Autodesk Inventor part; units mm, degrees
ref_plane "YZ Plane" through (0, 0, 0) normal (1, 0, 0) x (0, 1, 0)
ref_plane "XZ Plane" through (0, 0, 0) normal (0, 1, 0) x (-1, 0, 0)
ref_plane "XY Plane" through (0, 0, 0) normal (0, 0, 1) x (1, 0, 0)
ref_plane "Work Plane1" through (0, 0, 0) normal (0, 0, 1) x (1, 0, 0)
ref_plane "Work Plane2" through (0, 0, -10) normal (0, 0, 1) x (1, 0, 0)
sketch "Sketch1" plane through (0, 0, -10) normal (0, 0, 1) x (1, 0, 0)
  circle A0 centre (14.95, 17.4977) radius 7.15
  line L0 (0, 2.471) -> (29.9, 2.471)
  line L1 (0, 2.471) -> (0, 18.471)
  line L2 (0, 18.471) -> (-2, 18.471)
  line L3 (-2, 18.471) -> (-2, -1.5)
  line L4 (29.9, -1.5) -> (-2, -1.5)
  line L5 (29.9, -1.5) -> (29.9, 2.471)
  line L6 (4.95, 2.471) -> (24.95, 2.471)
  line L7 (24.95, 2.471) -> (24.95, 27.471)
  line L8 (24.95, 27.471) -> (4.95, 27.471)
  line L9 (4.95, 27.471) -> (4.95, 2.471)
  circle A1 centre (14.95, 17.4977) radius 8.1
  point P0 (0, 0)
  dimension "d6" = 20
  dimension "d7" = 25
  dimension "d8" = 10
  dimension "d23" = 16.2
extrude "Extrusion1" add sketch "Sketch1" against normal blind 30 contours L9 L8 L7 L0
sketch "Sketch2" plane through (4.95, 2.471, -10) normal (0, -1, 0) x (1, 0, 0)
  circle A0 centre (18.15, -13.73) radius 2.45
  circle A1 centre (1.85, -13.73) radius 2.75
  circle A2 centre (18.15, -13.73) radius 1.45
  circle A3 centre (1.85, -13.73) radius 1.45
  point P0 (-4.95, 10)
  dimension "d10" = 2.9
  dimension "d11" = 2.9
extrude "Extrusion2" cut sketch "Sketch2" against normal through all contours A2 | A3
chamfer "Chamfer1" distance 7 angle 45 2 edges at (24.95, 27.471, -25) (4.95, 27.471, -25)
sketch "Sketch3" plane through (11.95, 27.471, -10) normal (0, 1, 0) x (1, 0, 0)
  line L0 (0, 0) -> (0, 30)
  line L1 (6, 0) -> (0, 0)
  line L2 (6, 30) -> (6, 0)
  line L3 (0, 30) -> (6, 30)
  circle A0 centre (2, 5.2757) radius 1.45
  circle A1 centre (2, 26.8475) radius 1.45
  point P0 (-11.95, -10)
  dimension "d17" = 2.9
  dimension "d18" = 2.9
extrude "Extrusion3" cut sketch "Sketch3" against normal blind 10 contours A0 | A1
ref_plane "Work Plane3" through (0, 27.471, -10) normal (0, -0.7071068, 0.7071068) x (1, 0, 0)
ref_plane "Work Plane4" through (11.95, 27.471, -10) normal (0, 0.7071068, 0.7071068) x (1, 0, 0)
ref_plane "Work Plane5" through (14.95, 2.471, -10) normal (1, 0, 0) x (0, 0, -1)
sketch "Sketch5" plane through (14.95, 2.471, -10) normal (1, 0, 0) x (0, 0, -1)
  line L0 (0, 23.1268) -> (30, 23.1268)
  line L1 (0, 6.9268) -> (30, 6.9268)
  line L2 (0, 23.1268) -> (-4.2183, 23.1268)
  line L3 (-4.2183, 23.1268) -> (24.7731, 52.1181)
  line L4 (24.7731, 52.1181) -> (24.7731, 23.1268)
  point P0 (-10, -2.471)
  dimension "d21" = 41
  dimension "d22" = 45
properties part number "cellSTORM_v5_bluelaser_adapter"
Can you work these out from the model? Positions are in its coordinate system, mm. A direction names the side the tool comes from. Round coordinates to 2 decimals unless told otherwise and drop trailing zeros. Loops run counter-clockwise (first coordinate to the right, second up) from the corner with the lowest first, then second, coordinate; pieces in that order, holes last. Notation, with made-up numbers: M 68,52.5 L 93,52.5 A16 cw 93,78.5 Z; hole C -25.75,89 d3. An arc over 180 degrees is marked long. Answer in a Markdown table with one row per item.
1. Please list where these lines run through material, in increasing order: line 1 (Z direction, x = 13.95, y = 25.8); line 2 (Y direction, x = 15.25, z = -17.5); line 3 (X direction, y = 11, z = -23). Write a range as from..to.
Established:
| item | result |
|---|---|
| line 1 | -40..-38.3, -35.4..-16.73, -13.83..-10 |
| line 2 | 2.47..9.4, 25.59..27.47 |
| line 3 | 4.95..5.55, 8.05..10.11, 19.79..21.85, 24.35..24.95 |
2. If we section it at B-B, the plane x = 13.5: Please give me the cut outline in (y, z).
Established:
| item | result |
|---|---|
| outline | M 2.47,-40 L 9.53,-40 L 9.53,-10 L 2.47,-10 Z; M 25.47,-40 L 27.47,-40 L 27.47,-38.23 L 25.47,-38.23 Z; M 25.47,-35.47 L 27.47,-35.47 L 27.47,-16.65 L 25.47,-16.65 Z; M 25.47,-13.9 L 27.47,-13.9 L 27.47,-10 L 25.47,-10 Z |
3. If we section it at A-A, the plane y = 10: Please give me the cut outline in (x, z), plus the area to 3 significant figures.
Established:
| item | result |
|---|---|
| outline | M 4.95,-40 L 11.88,-40 L 11.88,-10 L 4.95,-10 Z; M 18.02,-40 L 24.95,-40 L 24.95,-10 L 18.02,-10 Z; hole C 6.8,-23.73 d2.9; hole C 23.1,-23.73 d2.9 |
| area | 403 mm² |
4. I'm going to push flat-ended pins straight in: pin 1 Ø4 at (x, z) = (13.95, -36.85) entering from +Y; pin 2 Ø9.5 at (x, y) = (14.95, 17.5) entering from +Z; pin 3 Ø4.5 at (x, z) = (23.1, -23.73) entering from +Y; pin 4 Ø1.7 at (x, z) = (13.95, -15.28) entering from +Y. Where does each tip first touch, or does it pass through?
Established:
| item | result |
|---|---|
| pin 1 | y = 27.47 |
| pin 2 | through |
| pin 3 | y = 24.57 |
| pin 4 | y = 9.61 |
5. On a 3-axis mill with a long thin cutter (end or side, diameter ignored), from which of +Z, -Z, +X, -X, +Y, -Y can I reach the whole of each face in a straight line? I mean faces 1 (the face through (24.95, 11, -25)), 2 (the face through (12.5, 26.4, -36.9)). Say none if no direction works.
Established:
| item | result |
|---|---|
| face 1 | +Z, -Z, +X, +Y, -Y |
| face 2 | +Y |
6. If we section it at C-C, the plane y = 18.5: Please give me the cut outline in (x, z).
Established:
| item | result |
|---|---|
| outline | M 4.95,-40 L 6.91,-40 L 6.91,-25.18 A1.45 cw long 6.91,-22.28 L 6.91,-10 L 4.95,-10 Z; M 22.99,-40 L 24.95,-40 L 24.95,-10 L 22.99,-10 L 22.99,-22.28 A1.45 cw long 22.99,-25.18 Z |
7. Thinking about a two-plate mould opening in X: for faces 3 (the face through (12.5, 26.4, -15.3)), 4 (the face through (21.4, 24.02, -24.79)), 5 (the face through (15, 27.471, -25)), which applies, pulls with the +X half, pulls with the -X half, needs draft (parallel to the pull), parting line crosses it, or undercut?
Established:
| item | result |
|---|---|
| face 3 | undercut |
| face 4 | pulls with the +X half |
| face 5 | needs draft |
8. If we section it at D-D, the plane z = -23.73: Please give me the cut outline in (x, y).
Established:
| item | result |
|---|---|
| outline | M 4.95,2.47 L 5.35,2.47 L 5.35,20.87 L 4.95,20.47 Z; M 8.25,2.47 L 21.65,2.47 L 21.65,12.95 A8.1 cw 8.25,12.95 Z; M 8.25,22.05 A8.1 cw 21.65,22.05 L 21.65,23.77 L 17.95,27.47 L 11.95,27.47 L 8.25,23.77 Z; M 24.55,2.47 L 24.95,2.47 L 24.95,20.47 L 24.55,20.87 Z |
